```python
from build123d import *

# Parameters (mm, degrees)
SKETCH_1_R      = 1.6
SKETCH_1_W      = 3
SKETCH_1_H      = 10
EXTRUDE_1_DEPTH = 3


with BuildPart() as part:
    # 草图1 → 凸台-拉伸1 (new body)
    with BuildSketch(Plane.XY):
        Polygon((32, 0), (44, 0), (56, 0), (56, -3), (76, -3), (76, 0), (88, 0), (91, 0), (91, 30), (88, 30), (0, 30), (-3, 30), (-3, 0), (0, 0), (12, 0), (12, -3), (32, -3), align=None)
        with Locations((30, 4)):
            Circle(SKETCH_1_R, mode=Mode.SUBTRACT)
        with Locations((9.5, 10)):
            Rectangle(SKETCH_1_W, SKETCH_1_H, mode=Mode.SUBTRACT)
        with BuildLine():
            ThreePointArc((59.6, 4), (58, 2.4), (56.4, 4))
            ThreePointArc((56.4, 4), (58, 5.6), (59.6, 4))
        make_face(mode=Mode.SUBTRACT)
        with Locations((78.5, 10)):
            Rectangle(SKETCH_1_W, SKETCH_1_H, mode=Mode.SUBTRACT)
        Polygon((0, 15), (0, 23), (3, 23), (3, 15), (3, 7), (0, 7), align=None, mode=Mode.SUBTRACT)
        Polygon((85, 23), (88, 23), (88, 15), (88, 7), (85, 7), (85, 15), align=None, mode=Mode.SUBTRACT)
    extrude(amount=EXTRUDE_1_DEPTH)


solid = part.part
```
Work out the finished part from the listing and answer in its coordinate system (mm). A direction names the side the tool comes from. Round coordinates to 2 decimals unless told otherwise and drop trailing zeros. Write each loop counter-clockwise with the first axis right and the second up, starting at its lowest first coordinate (ties: lowest second). Pieces come first, ordered by that corner, then holes. Notation, with made-up numbers: (87, -36.5) -> (111, -36.5) arc R18 ccw to (111, -23.5) -> close; hole circle Ø1 at (-20.75, 21.5). An arc over 180 degrees is marked (long way). Write each question's results on one line, items separated by ' | '.
Q1. Determine the mould class of faces 4 (the flat face through (4, 0, 1)), 5 (the flat face through (1, 23, 1)), 6 (the flat face through (43, 14, 3)) for opening direction Y: released by +Y, released by -Y, zero draft, split by the parting line, or undercut.
Data:
face 4: released by -Y | face 5: undercut | face 6: zero draft
Q2. Section D-D, the plane x = 30 is taken. Write down the section's boundary in (y, z).
Data:
outline: (-3, 0) -> (2.4, 0) -> (2.4, 3) -> (-3, 3) -> close; (5.6, 0) -> (30, 0) -> (30, 3) -> (5.6, 3) -> close
Q3. Straight lines are drawn through the part: line 1 along X through (y, z) = (9.5, 1.3); line 2 along X through (y, z) = (16.5, 2.75); line 3 along Y through (x, z) = (30, 1.55). For each, find the intervals that lie inside material, in ascending order. Write a range as [from, to].
Data:
line 1: [-3, 0], [3, 8], [11, 77], [80, 85], [88, 91] | line 2: [-3, 0], [3, 85], [88, 91] | line 3: [-3, 2.4], [5.6, 30]
Q4. Flat-ended cylindrical pins translate along their axes: P1, Ø1.5, axis at y = -1.5, z = 1, coming from the +X side; P2, Ø2, axis at x = 9.5, y = 22, coming from the -Z side. Find the tip coordinate at first contact, or state that the pin passes through.
Data:
P1: x = 76 | P2: z = 0
Q5. Section A-A, the plane y = 4 is taken. Write down the section's boundary in (x, z).
Data:
outline: (-3, 0) -> (28.4, 0) -> (28.4, 3) -> (-3, 3) -> close; (31.6, 0) -> (56.4, 0) -> (56.4, 3) -> (31.6, 3) -> close; (59.6, 0) -> (91, 0) -> (91, 3) -> (59.6, 3) -> close
Q6. Which of the six approach directions +Z, -Z, +X, -X, +Y, -Y give full straight-line access (tool end or side, diameter ignored) to faces 1 (the flat face through (56, -1, 1)), 2 (the flat face through (0, 15, 1)), 3 (the flat face through (66, -3, 1))?
Data:
face 1: +Z, -Z, -Y | face 2: +Z, -Z | face 3: +Z, -Z, +X, -X, -Y
Q7. Section C-C, the plane y = 12.5 is taken. Write down the section's boundary in (x, z).
Data:
outline: (-3, 0) -> (0, 0) -> (0, 3) -> (-3, 3) -> close; (3, 0) -> (8, 0) -> (8, 3) -> (3, 3) -> close; (11, 0) -> (77, 0) -> (77, 3) -> (11, 3) -> close; (80, 0) -> (85, 0) -> (85, 3) -> (80, 3) -> close; (88, 0) -> (91, 0) -> (91, 3) -> (88, 3) -> close
Q8. Section B-B, the plane z = 0.9 is taken. Give the number of separate pieces and of enclosed holes in the cut face, then the cut area to 3 significant figures.
Data:
separate pieces: 1 | enclosed holes: 6 | area: 2,770 mm^2
